Autodesk Inventor part; units mm, degrees
ref_plane "YZ Plane" through (0, 0, 0) normal (1, 0, 0) x (0, 1, 0)
ref_plane "XZ Plane" through (0, 0, 0) normal (0, 1, 0) x (-1, 0, 0)
ref_plane "XY Plane" through (0, 0, 0) normal (0, 0, 1) x (1, 0, 0)
sketch "Sketch1" plane through (0, 0, 0) normal (0, 0, 1) x (1, 0, 0)
  line L0 (0, 0) -> (42, 0)
  line L1 (42, 0) -> (42, 42)
  line L2 (42, 42) -> (0, 42)
  line L3 (0, 42) -> (0, 0)
  line L4 (5, 37) -> (37, 37) construction
  line L5 (37, 37) -> (37, 5) construction
  line L6 (37, 5) -> (5, 5) construction
  line L7 (5, 5) -> (5, 37) construction
  circle A0 centre (5, 37) radius 1.5
  circle A1 centre (37, 37) radius 1.5
  circle A2 centre (37, 5) radius 1.5
  circle A3 centre (5, 5) radius 1.5
  circle A4 centre (21, 21) radius 2.5
  point P0 (21, 42)
  point P1 (42, 21)
  dimension "d0" = 42
  dimension "d1" = 42
  dimension "d2" = 32
  dimension "d3" = 3
  dimension "d4" = 3
  dimension "d5" = 3
  dimension "d6" = 3
  dimension "d9" = 5
extrude "Extrusion1" add sketch "Sketch1" along normal blind 50
chamfer "Chamfer1" distance 3 angle 45 4 edges at (42, 42, 25) (42, 0, 25) (0, 0, 25) (0, 42, 25)
sketch "Sketch2" plane through (0, 0, 50) normal (0, 0, 1) x (1, 0, 0)
  circle A0 centre (21, 21) radius 2.5 construction
  circle A1 centre (21, 21) radius 10
  point P0 (0, 0)
  dimension "d13" = 20
sketch "Sketch3" plane through (0, 0, 50) normal (0, 0, 1) x (1, 0, 0)
  circle A0 centre (21, 21) radius 2.5
  point P0 (0, 0)
extrude "Extrusion2" add sketch "Sketch3" along normal blind 25
extrude "Extrusion3" add sketch "Sketch2" along normal blind 2
properties part number "NEMA42"
Check sheet for the modelled part. Datum: model origin and axes. Units: mm. A direction names the side the tool comes from. Give positions to 0.01 mm unless a question says otherwise; leave off trailing zeros. Loops run counter-clockwise (first coordinate to the right, second up) from the corner with the lowest first, then second, coordinate; pieces in that order, holes last. Notation, with made-up numbers: M -0.5,86.25 L 18.5,86.25 A15 ccw 18.5,101.25 Z; hole C -23,67 d7. An arc over 180 degrees is marked long. Answer as a JSON object with one key per item and string values. Group by question number.
Q1. Cross-section at D-D on x = 13. Record the cut outline in (y, z).
Q2. Cross-section at C-C on z = 42. Record the cut outline in (x, y), then the cut area to 3 significant figures.
Q3. Release check for a two-part mould opening along Y. For faces 4 (the flat face through (40, 1, 25)), 5 (the flat face through (16, 21, 0)), 6 (the cylindrical face through (35.8, 5.9, 24.6)), 7 (the flat face through (41, 40, 25)) record: released by +Y, released by -Y, zero draft, split by the parting line, or undercut.
Q4. Material ranges on line 1 along Y through (x, z) = (5, 27.5); line 2 along Z through (x, y) = (32.5, 21); line 3 along Z through (x, y) = (18.5, 20), recorded low to high. Write a range as [from, to].
Q5. Go/stop test with flat-tipped pins: P1, Ø1, axis at x = 8.5, y = 18, coming from the +Z side; P2, Ø1.5, axis at x = 21, y = 22, coming from the -Z side; P3, Ø5, axis at x = 13.5, y = 24.5, coming from the +Z side. Record where each tip stops, or that it passes through.
Q6. Cross-section at A-A on x = 37. Record the cut outline in (y, z).
Q7. Access from +Z, -Z, +X, -X, +Y, -Y to the whole of each face (thin tool, end or side, straight path). Record for faces 1 (the flat face through (30, 26, 50)), 2 (the flat face through (21, 21, 75)), 3 (the cylindrical face through (18.5, 20.9, 24.6)).
Evaluation:
{
 "1": {"outline": "M 0,0 L 42,0 L 42,50 L 27,50 L 27,52 L 15,52 L 15,50 L 0,50 Z"},
 "2": {"outline": "M 0,3 L 3,0 L 39,0 L 42,3 L 42,39 L 39,42 L 3,42 L 0,39 Z; hole C 5,5 d3; hole C 5,37 d3; hole C 21,21 d5; hole C 37,5 d3; hole C 37,37 d3", "area": "1,700 mm2"},
 "3": {"face 4": "released by -Y", "face 5": "zero draft", "face 6": "undercut", "face 7": "released by +Y"},
 "4": {"line 1": "y = [0, 3.5], [6.5, 35.5], [38.5, 42]", "line 2": "z = [0, 50]", "line 3": "z = [0, 52]"},
 "5": {"P1": "stops at z = 50", "P2": "stops at z = 50", "P3": "stops at z = 52"},
 "6": {"outline": "M 0,0 L 3.5,0 L 3.5,50 L 0,50 Z; M 6.5,0 L 35.5,0 L 35.5,50 L 6.5,50 Z; M 38.5,0 L 42,0 L 42,50 L 38.5,50 Z"},
 "7": {"face 1": "+Z", "face 2": "+Z, +X, -X, +Y, -Y", "face 3": "-Z"}
}
